Design review of the part built by this model. Coordinates are the model's own, in mm. Give positions to 0.01 mm unless a question says otherwise; leave off trailing zeros. Order: outer loops, then holes, each group sorted by start corner. A loop starts at its lowest first (then second) coordinate and runs counter-clockwise, first axis right, second up. Notation, with made-up numbers: (22, -35.75) -> (64, -35.75) arc R15 cw to (64, -15.75) -> close; hole circle Ø8 at (23.5, -31.75). An arc over 180 degrees is marked (long way). Use a Markdown table: item, result. Add a question column.
```python
from build123d import *

# Parameters (mm, degrees)
SKETCH1_W           = 205
SKETCH1_H           = 42
BOSS_EXTRUDE1_DEPTH = 6.35
SKETCH4_R           = 11
CUT_EXTRUDE3_DEPTH  = 7.35
CHAMFER1_SIZE       = 5
SKETCH5_R           = 11
CUT_EXTRUDE4_DEPTH  = 25
SKETCH13_R          = 11
SKETCH13_R_2        = 2.286
CUT_EXTRUDE12_DEPTH = 10


with BuildPart() as part:
    # Sketch1 → Boss-Extrude1 (new body)
    with BuildSketch(Plane.XY):
        Rectangle(SKETCH1_W, SKETCH1_H)
    extrude(amount=BOSS_EXTRUDE1_DEPTH)

    # Sketch4 → Cut-Extrude3 (cut, through all)
    with BuildSketch(Plane.XY.offset(6.35)):
        with Locations((-78.5, 0)):
            Circle(SKETCH4_R)
    extrude(amount=-CUT_EXTRUDE3_DEPTH, mode=Mode.SUBTRACT)

    # Chamfer1
    chamfer1_edges = [part.edges().sort_by_distance(p)[0] for p in [
        (102.5, -21, 3.175),
        (-102.5, -21, 3.175),
        (-102.5, 21, 3.175),
        (102.5, 21, 3.175),
    ]]
    chamfer(chamfer1_edges, length=CHAMFER1_SIZE)

    # Sketch5 → Cut-Extrude4 (cut)
    with BuildSketch(Plane.XY.offset(6.35)):
        with Locations((79.5, 0)):
            Circle(SKETCH5_R)
    extrude(amount=-CUT_EXTRUDE4_DEPTH, mode=Mode.SUBTRACT)

    # Sketch13 → Cut-Extrude12 (cut)
    with BuildSketch(Plane.XY.offset(6.35)):
        Polygon((-47.5, -16), (-47.5, 16), (-42.5, 21), (-97.5, 21), (-102.5, 16), (-102.5, -16), (-97.5, -21), (-42.5, -21), align=None)
        with Locations((-78.5, 0)):
            Circle(SKETCH13_R, mode=Mode.SUBTRACT)
        with Locations((-27.5, 10)):
            Circle(SKETCH13_R_2)
        with Locations((-12.5, 10)):
            Circle(SKETCH13_R_2)
        with Locations((-12.5, -10)):
            Circle(SKETCH13_R_2)
        with Locations((-27.5, -10)):
            Circle(SKETCH13_R_2)
        with Locations((2.5, 10)):
            Circle(SKETCH13_R_2)
        with Locations((17.5, 10)):
            Circle(SKETCH13_R_2)
        with Locations((17.5, -10)):
            Circle(SKETCH13_R_2)
        with Locations((2.5, -10)):
            Circle(SKETCH13_R_2)
    extrude(amount=-CUT_EXTRUDE12_DEPTH, mode=Mode.SUBTRACT)


solid = part.part
```
1) The part is to be moulded in two halves that separate along X. For faces 1 (the cylindrical face through (19.68, 10.69, 3.22)), 2 (the flat face through (102.5, 0, 3)), 3 (the flat face through (-47.5, 0, 3)), 4 (the flat face through (26, 0, 0)), say which applies: +X half, -X half, draft (parallel to the pull), parting line (faces both ways), or undercut.
2) Insertion check: pin 1 (2.5 mm diameter, centred on x = 17.5, y = -10, fed in from -Z). The pin has a flat end and moves straight along its axis. Give the tip position at first contact, or say it passes through.
3) Add section C-C (x = 79.5). Give the boundary of the cut face in (y, z).
4) Add section A-A (x = -12.5). Give the boundary of the cut face in (y, z).
5) Add section B-B (z = 5). Give the number of separate pieces and of enclosed holes in the cut face, then the cut area to 3 significant figures.
6) For L1, parallel to Y at x = -12.5, z = 2.75; L2, parallel to Y at x = 18, z = 2.75; L3, parallel to X at y = 9, z = 1.5, list the stretches that pass through material, from the lowest coordinate up. Write a range as [from, to].
7) Add section D-D (y = 0). Give the boundary of the cut face in (x, z), then the cut area to 3 significant figures.
Worked answers:
| question | item | result |
|---|---|---|
| 1 | face 1 | undercut |
| 1 | face 2 | +X half |
| 1 | face 3 | -X half |
| 1 | face 4 | draft |
| 2 | pin 1 | through |
| 3 | outline | (-21, 0) -> (-11, 0) -> (-11, 6.35) -> (-21, 6.35) -> close; (11, 0) -> (21, 0) -> (21, 6.35) -> (11, 6.35) -> close |
| 4 | outline | (-21, 0) -> (-12.29, 0) -> (-12.29, 6.35) -> (-21, 6.35) -> close; (-7.71, 0) -> (7.71, 0) -> (7.71, 6.35) -> (-7.71, 6.35) -> close; (12.29, 0) -> (21, 0) -> (21, 6.35) -> (12.29, 6.35) -> close |
| 5 | separate pieces | 1 |
| 5 | enclosed holes | 9 |
| 5 | area | 5,740 mm^2 |
| 6 | L1 | [-21, -12.29], [-7.71, 7.71], [12.29, 21] |
| 6 | L2 | [-21, -12.23], [-7.77, 7.77], [12.23, 21] |
| 6 | L3 | [-47.5, -29.56], [-25.44, -14.56], [-10.44, 0.44], [4.56, 15.44], [19.56, 73.18], [85.82, 102.5] |
| 7 | outline | (-47.5, 0) -> (68.5, 0) -> (68.5, 6.35) -> (-47.5, 6.35) -> close; (90.5, 0) -> (102.5, 0) -> (102.5, 6.35) -> (90.5, 6.35) -> close |
| 7 | area | 813 mm^2 |
